from build123d import *

# Parameters (mm, degrees)
ESQUISSE2_R        = 1.25
BOSS_EXTRU_1_DEPTH = 2
ESQUISSE3_R        = 2.5
ESQUISSE3_R_2      = 1.25
BOSS_EXTRU_2_DEPTH = 4.2


with BuildPart() as part:
    # Esquisse1 → Révolution1 (revolve)
    with BuildSketch(Plane.XY, mode=Mode.PRIVATE) as r_volution1_sk:
        Polygon((1.25, 0), (1.25, 5.8), (3.5, 5.8), (3.5, 3.8), (2.5, 3.8), (2.5, 0), align=None)
    revolve(r_volution1_sk.sketch.rotate(Axis((0, 0, 0), (0, 1, 0)), 90), axis=Axis((0, 0, 0), (0, 1, 0)))

    # Esquisse2 → Boss.-Extru.1 (add)
    with BuildSketch(Plane.XZ):
        Polygon((4, 2.309401077), (0, 4.618802154), (-4, 2.309401077), (-4, -2.309401077), (0, -4.618802154), (4, -2.309401077), align=None)
        with Locations(Location((0, 0, 0), (0, 0, 270))):
            Circle(ESQUISSE2_R, mode=Mode.SUBTRACT)
    extrude(amount=BOSS_EXTRU_1_DEPTH)

    # Esquisse3 → Boss.-Extru.2 (add)
    with BuildSketch(Plane.XZ.offset(2)):
        with Locations(Location((0, 0, 0), (0, 0, 270))):
            Circle(ESQUISSE3_R)
        with Locations(Location((0, 0, 0), (0, 0, 270))):
            Circle(ESQUISSE3_R_2, mode=Mode.SUBTRACT)
    extrude(amount=BOSS_EXTRU_2_DEPTH)


solid = part.part
Could you check a few things on this model? Use its own coordinates, in mm. A direction names the side the tool comes from. Round coordinates to 2 decimals unless told otherwise and drop trailing zeros. Write each loop counter-clockwise with the first axis right and the second up, starting at its lowest first coordinate (ties: lowest second). Pieces come first, ordered by that corner, then holes. Notation, with made-up numbers: (-28, 87) -> (-22, 87) arc R27 ccw to (-22, 120) -> close; hole circle Ø10 at (-4.75, 61). An arc over 180 degrees is marked (long way). Use a Markdown table: item, result.
1. Please list where these lines run through material, in increasing order: probe 1 along Y at (x, z) = (-2.25, 1.25); probe 2 along X at (y, z) = (-3.8, 0); probe 3 along X at (y, z) = (-0.5, 0).
Answer key:
| item | result |
|---|---|
| probe 1 | y = -2 to 0, 3.8 to 5.8 |
| probe 2 | x = -2.5 to -1.25, 1.25 to 2.5 |
| probe 3 | x = -4 to -1.25, 1.25 to 4 |
2. If we section it at C-C (x = 2.25): List the corners of the cut face in (y, z) for me.
Answer key:
| item | result |
|---|---|
| outline | (-6.2, -1.09) -> (-2, -1.09) -> (-2, -3.32) -> (0, -3.32) -> (0, -1.09) -> (3.8, -1.09) -> (3.8, -2.68) -> (5.8, -2.68) -> (5.8, 2.68) -> (3.8, 2.68) -> (3.8, 1.09) -> (0, 1.09) -> (0, 3.32) -> (-2, 3.32) -> (-2, 1.09) -> (-6.2, 1.09) -> close |
3. For pin 1 Ø3 at (x, y) = (1.5, 4.5) entering from -Z, with a flat end and sliding along its axis, tell me the tip position at first contact or that it passes through.
Answer key:
| item | result |
|---|---|
| pin 1 | stops at z = -3.5 |
4. If we section it at A-A (y = -1): List the corners of the cut face in (x, z) for me, then the cut area to 3 significant figures.
Answer key:
| item | result |
|---|---|
| outline | (-4, -2.31) -> (0, -4.62) -> (4, -2.31) -> (4, 2.31) -> (0, 4.62) -> (-4, 2.31) -> close; hole circle Ø2.5 at (0, 0) |
| area | 50.5 mm^2 |
5. If we section it at D-D (z = 0): List the corners of the cut face in (x, y) for me.
Answer key:
| item | result |
|---|---|
| outline | (-4, -2) -> (-2.5, -2) -> (-2.5, -6.2) -> (-1.25, -6.2) -> (-1.25, 5.8) -> (-3.5, 5.8) -> (-3.5, 3.8) -> (-2.5, 3.8) -> (-2.5, 0) -> (-4, 0) -> close; (1.25, -6.2) -> (2.5, -6.2) -> (2.5, -2) -> (4, -2) -> (4, 0) -> (2.5, 0) -> (2.5, 3.8) -> (3.5, 3.8) -> (3.5, 5.8) -> (1.25, 5.8) -> close |
6. We'd pull the mould along Y, two halves only. Please class faces 6 (the face through (-0.1, 1.9, 2.5)), 7 (the face through (2.028, -0.986, 3.448)), 8 (the face through (2, 0, -2)), 9 (the face through (1, -6.2, -1)): +Y half, -Y half, draft (parallel to the pull), parting line (faces both ways), or undercut.
Answer key:
| item | result |
|---|---|
| face 6 | undercut |
| face 7 | draft |
| face 8 | undercut |
| face 9 | -Y half |
7. If we section it at B-B (z = -2.75): List the corners of the cut face in (x, y) for me.
Answer key:
| item | result |
|---|---|
| outline | (-3.24, -2) -> (3.24, -2) -> (3.24, 0) -> (-3.24, 0) -> close; (-2.17, 3.8) -> (2.17, 3.8) -> (2.17, 5.8) -> (-2.17, 5.8) -> close |
8. Which directions (+Z, -Z, +X, -X, +Y, -Y) give clear straight access to the entire face, cutting with the end or side of a thin tool? Please do faces 1 (the face through (2, 3.8, -2)), 2 (the face through (-4, -1, 0)), 3 (the face through (4, -1, 0)), 4 (the face through (-2.44, -4.07, 0.54)), 5 (the face through (3.105, 4.786, -1.615)).
Answer key:
| item | result |
|---|---|
| face 1 | none |
| face 2 | +Z, -Z, -X, +Y, -Y |
| face 3 | +Z, -Z, +X, +Y, -Y |
| face 4 | -Y |
| face 5 | +Y |
